from build123d import *

# Parameters (mm, degrees)
SKETCH1_W           = 950
SKETCH1_H           = 110.864689034
BOSS_EXTRUDE1_DEPTH = 27.5
SKETCH2_R           = 47.5
CUT_EXTRUDE1_DEPTH  = 53
SKETCH3_R           = 32.5
CUT_EXTRUDE2_DEPTH  = 53
CHAMFER1_SIZE       = 5


with BuildPart() as part:
    # Sketch1 → Boss-Extrude1 (new, symmetric)
    with BuildSketch(Plane(origin=(0, 0, 0), x_dir=(1, 0, 0), z_dir=(0, 1, 0))):
        Rectangle(SKETCH1_W, SKETCH1_H)
    extrude(amount=BOSS_EXTRUDE1_DEPTH, both=True)

    # Sketch2 → Cut-Extrude1 (cut)
    with BuildSketch(Plane(origin=(0, 27.5, 0), x_dir=(1, 0, 0), z_dir=(0, 1, 0))):
        with Locations(Location((0, 0, 0), (0, 0, 270))):
            Circle(SKETCH2_R)
    extrude(amount=-CUT_EXTRUDE1_DEPTH, mode=Mode.SUBTRACT)

    # Sketch3 → Cut-Extrude2 (cut)
    with BuildSketch(Plane(origin=(0, -25.5, 0), x_dir=(1, 0, 0), z_dir=(0, 1, 0))):
        with Locations(Location((0, 0, 0), (0, 0, 270))):
            Circle(SKETCH3_R)
    extrude(amount=-CUT_EXTRUDE2_DEPTH, mode=Mode.SUBTRACT)

    # Chamfer1
    chamfer1_edges = [part.edges().sort_by_distance(p)[0] for p in [
        (0, 27.5, -55.432344517),
    ]]
    chamfer(chamfer1_edges, length=CHAMFER1_SIZE)


solid = part.part
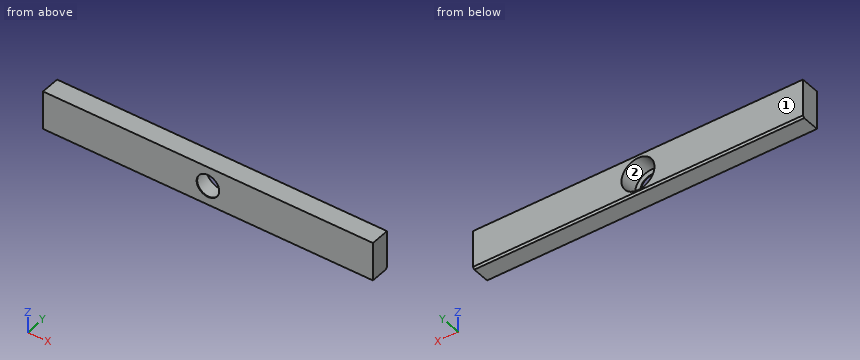
Work out the finished part from the listing and answer in its coordinate system (mm). Face numbers are marked on the shaded views. Give positions to 0.01 mm unless a question says otherwise; leave off trailing zeros. Loops run counter-clockwise (first coordinate to the right, second up) from the corner with the lowest first, then second, coordinate; pieces in that order, holes last. Notation, with made-up numbers: (87.5, 73) -> (145.5, 73) arc R20 cw to (145.5, 89) -> close; hole circle Ø10 at (8.25, 9.25). An arc over 180 degrees is marked (long way). Use a Markdown table: item, result. Add a question column.
1. Determine the mould class of the marked faces 1 and 2 for opening direction X: released by +X, released by -X, zero draft, split by the parting line, or undercut.
2. Find the intervals of material crossed by probe 1 along X at (y, z) = (-26, 0); probe 2 along X at (y, z) = (-5, 0); probe 3 along Y at (x, z) = (-34, 7.5), in increasing order.
3. Section A-A on x = 0 is taken. Determine the outline of the cut face in (y, z).
4. Section B-B on z = 0 is taken. Determine the outline of the cut face in (x, y).
5. Section C-C on y = -2.5 is taken. Determine the outline of the cut face in (x, z).
Results below:
| question | item | result |
|---|---|---|
| 1 | face 1 | zero draft |
| 1 | face 2 | undercut |
| 2 | probe 1 | x = -475 to -32.5, 32.5 to 475 |
| 2 | probe 2 | x = -475 to -47.5, 47.5 to 475 |
| 2 | probe 3 | y = -27.5 to -25.5 |
| 3 | outline | (-27.5, -55.43) -> (22.5, -55.43) -> (27.5, -50.43) -> (27.5, -47.5) -> (-25.5, -47.5) -> (-25.5, -32.5) -> (-27.5, -32.5) -> close; (-27.5, 32.5) -> (-25.5, 32.5) -> (-25.5, 47.5) -> (27.5, 47.5) -> (27.5, 55.43) -> (-27.5, 55.43) -> close |
| 4 | outline | (-475, -27.5) -> (-32.5, -27.5) -> (-32.5, -25.5) -> (-47.5, -25.5) -> (-47.5, 27.5) -> (-475, 27.5) -> close; (32.5, -27.5) -> (475, -27.5) -> (475, 27.5) -> (47.5, 27.5) -> (47.5, -25.5) -> (32.5, -25.5) -> close |
| 5 | outline | (-475, -55.43) -> (475, -55.43) -> (475, 55.43) -> (-475, 55.43) -> close; hole circle Ø95 at (0, 0) |
